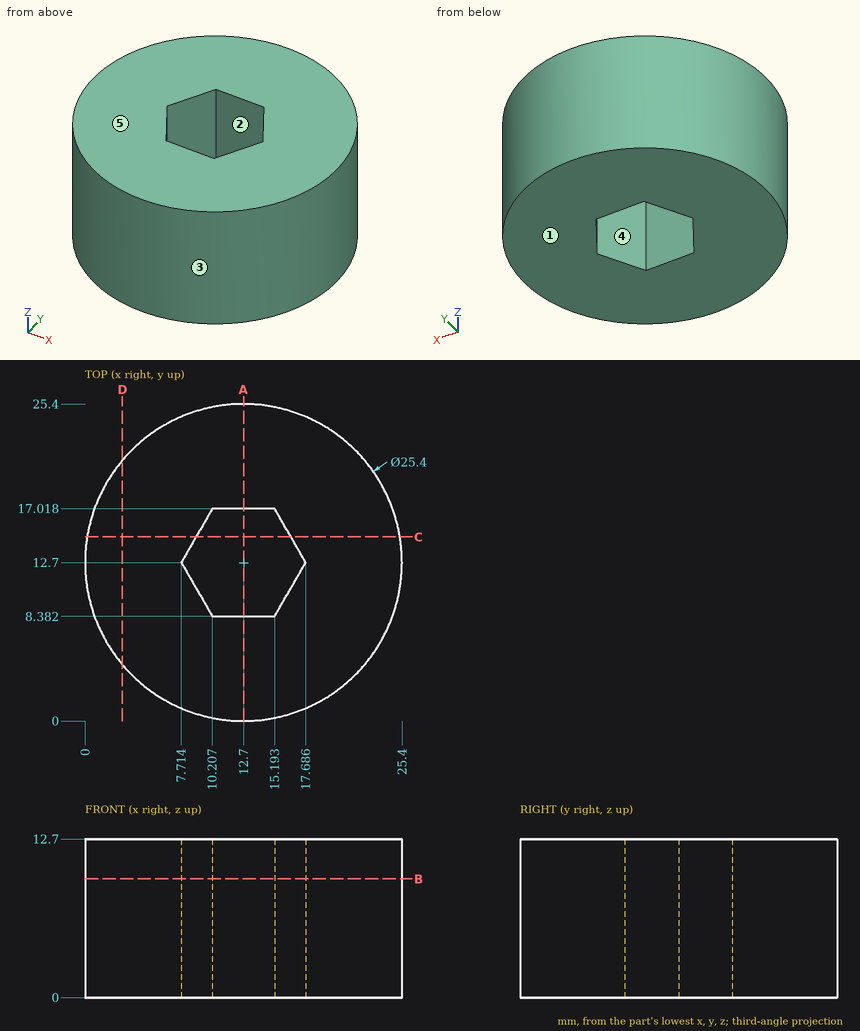
Input: dimensioned drawing with shaded views. Units: mm. Origin: part minimum x, y, z. A direction names the side the tool comes from. Give positions to 0.01 mm unless a question says otherwise; leave off trailing zeros. Write each loop counter-clockwise with the first axis right and the second up, starting at its lowest first coordinate (ties: lowest second). Pieces come first, ordered by that corner, then holes. Notation, with made-up numbers: (73, 55.5) - (116, 55.5) arc R23 cw to (116, 71.5) - close; hole circle Ø11 at (1, 4). An arc over 180 degrees is marked (long way). One line per item, written item: value. Start each with the question number.
Q1. Section query A-A, the plane x = 12.7. Return the cut outline in (y, z), then the cut area to 3 significant figures.
Q2. Draft query along Y for the marked faces 1, 2 and 3. Return one class per face: +Y half, -Y half, draft (parallel to the pull), parting line (faces both ways), or undercut.
Q3. Section query D-D, the plane x = 3. Return the cut outline in (y, z), then the cut area to 3 significant figures.
Q4. Section query B-B, the plane z = 9.5. Return the cut outline in (x, y).
Q5. Section query C-C, the plane y = 14.75. Return the cut outline in (x, z).
Q6. First-contact query: pin 1 Ø1.5 at (x, z) = (12, 6.5) entering from +Y; pin 2 Ø2 at (y, z) = (15.5, 3.5) entering from -X; pin 3 Ø5 at (x, z) = (8, 8) entering from +Y; pin 4 Ø6 at (x, z) = (4.5, 6) entering from -Y. Flat tips, straight axial feed; report the tip coordinate or a pass-through.
Q7. Material intervals for probe 1 along X at (y, z) = (11, 3.25); probe 2 along X at (y, z) = (11.5, 8); probe 3 along Y at (x, z) = (10.5, 0.75), sorted ascending. Write a range as from..to.
Q8. Set-up query: the marked faces 4 and 5. Return all of +Z, -Z, +X, -X, +Y, -Y with unobstructed straight access to the full face (end or side cutting, diameter ignored); none if empty.
Answer:
1. outline: (0, 0) - (8.38, 0) - (8.38, 12.7) - (0, 12.7) - close; (17.02, 0) - (25.4, 0) - (25.4, 12.7) - (17.02, 12.7) - close
1. area: 213 mm2
2. face 1: draft
2. face 2: undercut
2. face 3: parting line
3. outline: (4.5, 0) - (20.9, 0) - (20.9, 12.7) - (4.5, 12.7) - close
3. area: 208 mm2
4. outline: circle Ø25.4 at (12.7, 12.7); hole (7.71, 12.7) - (10.21, 8.38) - (15.19, 8.38) - (17.69, 12.7) - (15.19, 17.02) - (10.21, 17.02) - close
5. outline: (0.17, 0) - (8.9, 0) - (8.9, 12.7) - (0.17, 12.7) - close; (16.5, 0) - (25.23, 0) - (25.23, 12.7) - (16.5, 12.7) - close
6. pin 1: stops at y = 25.4
6. pin 2: stops at x = 0.13
6. pin 3: stops at y = 25.21
6. pin 4: stops at y = 1.11
7. probe 1: x = 0.11..8.7, 16.7..25.29
7. probe 2: x = 0.06..8.41, 16.99..25.34
7. probe 3: y = 0.19..8.38, 17.02..25.21
8. face 4: +Z, -Z
8. face 5: +Z, +X, -X, +Y, -Y
